Geometry check sheet. Reference: the model listing, model coordinates, mm. Face numbers are marked on the shaded views. A direction names the side the tool comes from. Round coordinates to 2 decimals unless told otherwise and drop trailing zeros. Loops run counter-clockwise (first coordinate to the right, second up) from the corner with the lowest first, then second, coordinate; pieces in that order, holes last. Notation, with made-up numbers: M -25,-33 L -9,-33 A37 cw -9,4 Z; hole C 70.5,14 d11. An arc over 180 degrees is marked long. Write item = value, one per line.
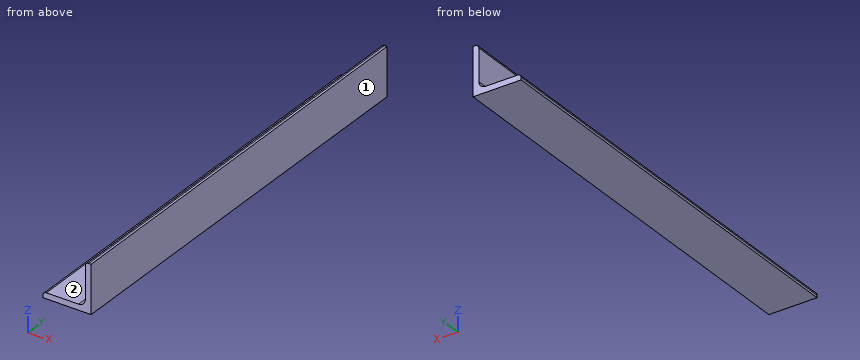
from build123d import *

# Parameters (mm, degrees)
BOSS_EXTRUDE1_DEPTH = 222.5


with BuildPart() as part:
    # Sketch1 → Boss-Extrude1 (new, symmetric)
    with BuildSketch(Plane(origin=(0, 0, 0), x_dir=(1, 0, 0), z_dir=(0, 1, 0))):
        with BuildLine():
            Line((0, 0), (-50, 0))
            Line((-50, 0), (-50, -2.5))
            ThreePointArc((-50, -2.5), (-48.974873734, -4.974873734), (-46.5, -6))
            Line((-46.5, -6), (-13, -6))
            ThreePointArc((-13, -6), (-8.050252532, -8.050252532), (-6, -13))
            Line((-6, -13), (-6, -46.5))
            ThreePointArc((-6, -46.5), (-4.974873734, -48.974873734), (-2.5, -50))
            Line((-2.5, -50), (0, -50))
            Line((0, -50), (0, 0))
        make_face()
    extrude(amount=BOSS_EXTRUDE1_DEPTH, both=True)


solid = part.part
(1) Sectioned sample at B-B on x = -20. Record the cut outline in (y, z).
Result set:
outline = M -222.5,0 L 222.5,0 L 222.5,6 L -222.5,6 Z
(2) Sectioned sample at A-A on y = 34. Record the cut outline in (x, z), then the cut area to 3 significant figures.
Result set:
outline = M -50,0 L 0,0 L 0,50 L -2.5,50 A3.5 ccw -6,46.5 L -6,13 A7 cw -13,6 L -46.5,6 A3.5 ccw -50,2.5 Z
area = 569 mm2
(3) Depth check by flat-ended pin: pin 1 Ø8 at (x, y) = (-38.5, 3) entering from +Z; pin 2 Ø4 at (y, z) = (5, 18) entering from -X; pin 3 Ø1.5 at (y, z) = (-103.5, 5.5) entering from -X. Enter the tip coordinate at first touch or a pass-through.
Result set:
pin_1 = 6
pin_2 = -6
pin_3 = -49.18
(4) Tool access check on the marked faces 1 and 2. Record the directions out of +Z, -Z, +X, -X, +Y, -Y that give a thin tool (end or side, any length) a straight path to the whole face; none if there is none.
Result set:
face_1 = +Z, -Z, +X, +Y, -Y
face_2 = +Z, -X, +Y, -Y
(5) Material ranges on line 1 along Z through (x, y) = (-33.5, -196.5); line 2 along X through (y, z) = (186, 32); line 3 along Z through (x, y) = (-8, 71), recorded low to high. Write a range as from..to.
Result set:
line_1 = 0..6
line_2 = -6..0
line_3 = 0..8.1
(6) Sectioned sample at C-C on z = 28. Record the cut outline in (x, y), then the cut area to 3 significant figures.
Result set:
outline = M -6,-222.5 L 0,-222.5 L 0,222.5 L -6,222.5 Z
area = 2,670 mm2
